Check sheet for the modelled part. Datum: model origin and axes. Units: mm. A direction names the side the tool comes from. Coordinates: 2 decimals unless noted, no trailing zeros. Order: outer loops, then holes, each group sorted by start corner. A loop starts at its lowest first (then second) coordinate and runs counter-clockwise, first axis right, second up.
1. Gauge pin test, flat ends, axial feed: pin 1 Ø1 at (y, z) = (17.5, 3.5) entering from -X; pin 2 Ø0.9 at (x, z) = (7.5, 3.5) entering from +Y; pin 3 Ø1.5 at (x, z) = (9, 3) entering from -Y. Record the tip position at first contact, or that the pin passes through.
2. Set-up check for faces 1 (the flat face through (8, 18.5, 4)), 2 (the cylindrical face through (9, 1, 2)): record each of +Z, -Z, +X, -X, +Y, -Y from which the full face is reachable in a straight line by a thin tool's end or side.
3. Draft check along Y on faces 3 (the cylindrical face through (9, 19, 2)), 4 (the flat face through (15.5, 10, 4)), 5 (the cylindrical face through (16, 10, 2)). Enter one of: released by +Y, released by -Y, zero draft, split by the parting line, or undercut.
4. Cross-section at C-C (z = 3.95). Enter the section's corners in (x, y), then the cut area to 3 significant figures.
5. Cross-section at D-D (z = 2.6). Enter the section's corners in (x, y).
6. Thickness scan on line 1 (Z direction, x = 7.25, y = 6); line 2 (Y direction, x = 11.75, z = 3.4); line 3 (X direction, y = 16, z = 3.7). Record the ranges inside material, lowest first.
```python
from build123d import *

# Parameters (mm, degrees)
F0_W     = 17
F0_H     = 20
F1_DEPTH = 5
F2_W     = 14.3
F2_H     = 17.3
F3_DEPTH = 3
F4_R     = 4.99999


# Not quite as in the source:
# - a fillet or chamfer is up to 0.001 mm smaller than in the source, because OpenCascade refuses the exact size


with BuildPart() as f1:
    # F0 (on Top) → F1 (new body)
    with BuildSketch(Plane.XY):
        with Locations((8.5, 10)):
            Rectangle(F0_W, F0_H)
    extrude(amount=F1_DEPTH)

    # F2 (on face) → F3 (cut)
    with BuildSketch(Plane.XY.offset(5)):
        with Locations((8.35, 9.85)):
            Rectangle(F2_W, F2_H)
    extrude(amount=-F3_DEPTH, mode=Mode.SUBTRACT)

    # F4 (radius 5 in the source; OpenCascade refuses exactly that, so slightly less here)
    f4_edges = [f1.edges().sort_by_distance(p)[0] for p in [
        (0, 10, 0),
        (8.5, 20, 0),
        (17, 10, 0),
        (8.5, 0, 0),
    ]]
    fillet(f4_edges, radius=F4_R)


solid = f1.part
```
Data:
1. pin 1: stops at x = 0.1
1. pin 2: stops at y = 19.89
1. pin 3: stops at y = 0.16
2. face 1: +Z
2. face 2: -Z, +X, -X, -Y
3. face 3: released by +Y
3. face 4: undercut
3. face 5: zero draft
4. outline: (0.11, 0.11) - (16.89, 0.11) - (16.89, 19.89) - (0.11, 19.89) - close; hole (1.2, 1.2) - (15.5, 1.2) - (15.5, 18.5) - (1.2, 18.5) - close
4. area: 84.4 mm2
5. outline: (0.61, 0.61) - (16.39, 0.61) - (16.39, 19.39) - (0.61, 19.39) - close; hole (1.2, 1.2) - (15.5, 1.2) - (15.5, 18.5) - (1.2, 18.5) - close
6. line 1: z = 0 to 2
6. line 2: y = 0.26 to 1.2, 18.5 to 19.74
6. line 3: x = 0.17 to 1.2, 15.5 to 16.83
